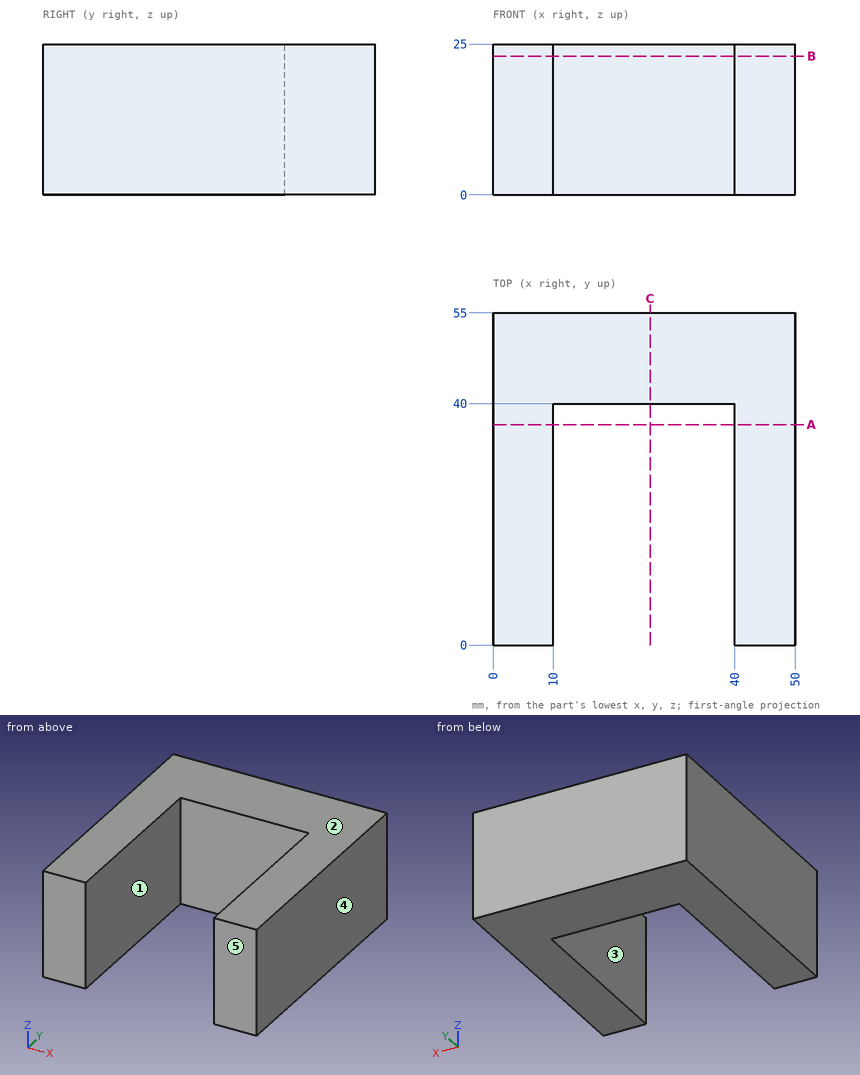
The drawing under review shows one solid part. Ordinate dimensions are in mm from its lowest x, y, z. A direction names the side the tool comes from. Coordinates: 2 decimals unless noted, no trailing zeros. Loops run counter-clockwise (first coordinate to the right, second up) from the corner with the lowest first, then second, coordinate; pieces in that order, holes last. Notation, with made-up numbers: (29, 72.5) - (79, 72.5) arc R22 ccw to (79, 81.5) - close; hole circle Ø4 at (15.5, -39.5). An arc over 180 degrees is marked (long way). Return JSON: item names as keys, results as strings.
Item 1: For line 1 (X direction, y = 11.5, z = 2); line 2 (Y direction, x = 15, z = 19.75), list the stretches that pass through material, from the lowest coordinate up.
Determined:
{"line 1": "x = 0 to 10, 40 to 50", "line 2": "y = 40 to 55"}
Item 2: Take a section at B-B (z = 23). Give the boundary of the cut face in (x, y).
Determined:
{"outline": "(0, 0) - (10, 0) - (10, 40) - (40, 40) - (40, 0) - (50, 0) - (50, 55) - (0, 55) - close"}
Item 3: Insertion check: pin 1 (1 mm diameter, centred on x = 13.5, z = 4.5, fed in from -Y). The pin has a flat end and moves straight along its axis. Give the tip position at first contact, or say it passes through.
Determined:
{"pin 1": "stops at y = 40"}
Item 4: Take a section at C-C (x = 26). Give the boundary of the cut face in (y, z).
Determined:
{"outline": "(40, 0) - (55, 0) - (55, 25) - (40, 25) - close"}
Item 5: Take a section at A-A (y = 36.5). Give the boundary of the cut face in (x, z), then the cut area to 3 significant figures.
Determined:
{"outline": "(0, 0) - (10, 0) - (10, 25) - (0, 25) - close; (40, 0) - (50, 0) - (50, 25) - (40, 25) - close", "area": "500 mm2"}
Item 6: Mouldability with a two-part tool opening along X and no side actions: class the marked faces 3, 4 and 5 as pulls with the +X half, pulls with the -X half, needs draft (parallel to the pull), parting line crosses it, or undercut.
Determined:
{"face 3": "undercut", "face 4": "pulls with the +X half", "face 5": "needs draft"}
Item 7: For the marked faces 1 and 2, list the 3-axis set-ups (+Z, -Z, +X, -X, +Y, -Y) from which the entire face can be reached by the end or side of a thin tool; tool diameter is ignored.
Determined:
{"face 1": "+Z, -Z, -Y", "face 2": "+Z, +X, -X, +Y, -Y"}
